Build history of the part. All positions in model axes, mm. Round coordinates to 2 decimals unless told otherwise and drop trailing zeros. Write each loop counter-clockwise with the first axis right and the second up, starting at its lowest first coordinate (ties: lowest second). Pieces come first, ordered by that corner, then holes. Notation, with made-up numbers: M 87,48 L 92,48 A14 ccw 92,59 Z; hole C 30,-32 d11. An arc over 180 degrees is marked long. Write item = value, one per line.
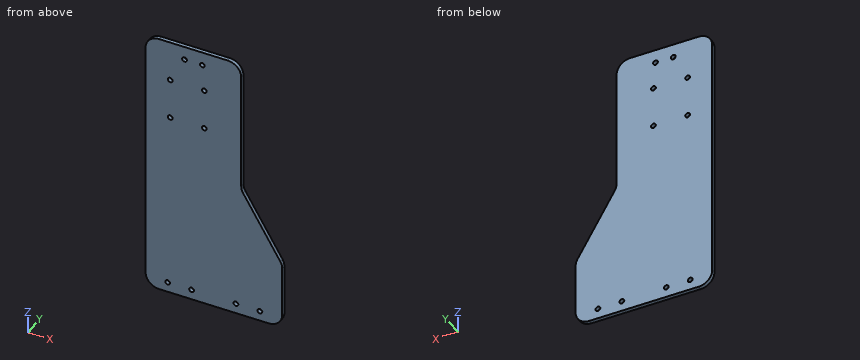
from build123d import *

# Parameters (mm, degrees)
SKETCH_1_W          = 100
SKETCH_1_H          = 200
EXTRUDE_1_DEPTH     = 3
CUT_EXTRUDE_1_DEPTH = 10
FILLET_2_R          = 10
SKETCH_4_R          = 1.75
CUT_EXTRUDE_2_DEPTH = 21
SKETCH_5_R          = 1.75
CUT_EXTRUDE_3_DEPTH = 4
SKETCH_7_R          = 1.75
CUT_EXTRUDE_4_DEPTH = 4


with BuildPart() as part:
    # 草图1 → 凸台-拉伸1 (new body)
    with BuildSketch(Plane(origin=(0, 0, 0), x_dir=(1, 0, 0), z_dir=(0, 1, 0))):
        Rectangle(SKETCH_1_W, SKETCH_1_H)
    extrude(amount=EXTRUDE_1_DEPTH)

    # 草图3 → 切除-拉伸1 (cut)
    with BuildSketch(Plane(origin=(0, 3, 0), x_dir=(1, 0, 0), z_dir=(0, 1, 0))):
        Polygon((20, -100), (20, 0), (50, 50), (50, -100), align=None)
    extrude(amount=-CUT_EXTRUDE_1_DEPTH, mode=Mode.SUBTRACT)

    # 圆角2
    fillet_2_edges = [part.edges().sort_by_distance(p)[0] for p in [
        (20, 1.5, 100),
        (20, 1.5, 0),
        (50, 1.5, -50),
        (-50, 1.5, 100),
        (-50, 1.5, -100),
        (50, 1.5, -100),
    ]]
    fillet(fillet_2_edges, radius=FILLET_2_R)

    # 草图4 → 切除-拉伸2 (cut)
    with BuildSketch(Plane(origin=(0, 3, 0), x_dir=(1, 0, 0), z_dir=(0, 1, 0))):
        with Locations(Location((33.647397187, 92.5, 0), (0, 0, 270))):
            Circle(SKETCH_4_R)
        with Locations(Location((16.132669012, 92.5, 0), (0, 0, 270))):
            Circle(SKETCH_4_R)
        with Locations(Location((-33.867330988, 92.5, 0), (0, 0, 270))):
            Circle(SKETCH_4_R)
        with Locations(Location((-16.352602813, 92.5, 0), (0, 0, 270))):
            Circle(SKETCH_4_R)
    extrude(amount=-CUT_EXTRUDE_2_DEPTH, mode=Mode.SUBTRACT)

    # 草图5 → 切除-拉伸3 (cut)
    with BuildSketch(Plane.XZ):
        with Locations(Location((-8.5, 90, 0), (0, 0, 270))):
            Circle(SKETCH_5_R)
        with Locations(Location((-21.5, 90, 0), (0, 0, 270))):
            Circle(SKETCH_5_R)
    extrude(amount=-CUT_EXTRUDE_3_DEPTH, mode=Mode.SUBTRACT)

    # 草图7 → 切除-拉伸4 (cut)
    with BuildSketch(Plane(origin=(0, 3, 0), x_dir=(1, 0, 0), z_dir=(0, 1, 0))):
        with Locations(Location((-32, -40, 0), (0, 0, 270))):
            Circle(SKETCH_7_R)
        with Locations(Location((-7, -40, 0), (0, 0, 270))):
            Circle(SKETCH_7_R)
        with Locations(Location((-7, -70, 0), (0, 0, 90))):
            Circle(SKETCH_7_R)
        with Locations(Location((-32, -70, 0), (0, 0, 90))):
            Circle(SKETCH_7_R)
    extrude(amount=-CUT_EXTRUDE_4_DEPTH, mode=Mode.SUBTRACT)


solid = part.part
1. Band-saw the part on A-A (y = 0.55). Count the separate pieces of the cut face and the enclosed holes in it, plus the area to 3 significant figures.
Responses:
separate_pieces = 1
enclosed_holes = 10
area = 16,100 mm²
2. Band-saw the part on B-B (z = -44). List the corners of the cut face in (x, y).
Responses:
outline = M -50,0 L 46.4,0 L 46.4,3 L -50,3 Z
3. Flat gauge pins, fed straight in: pin 1 (3 mm diameter, centred on x = -8.5, z = 90, fed in from +Y); pin 2 (5.5 mm diameter, centred on x = -7, z = 40, fed in from +Y); pin 3 (1.5 mm diameter, centred on y = 2, z = 61.5, fed in from +X). Where does each tip first touch, or does it go through?
Responses:
pin_1 = through
pin_2 = 3
pin_3 = 20
4. Band-saw the part on C-C (z = 14). List the corners of the cut face in (x, y).
Responses:
outline = M -50,0 L 20,0 L 20,3 L -50,3 Z
5. Probe probe 1 along X at (y, z) = (1.2, 70); probe 2 along X at (y, z) = (1.5, -92.5); probe 3 along X at (y, z) = (2.6, 58). List the from-to ranges inside material, lowest first.
Responses:
probe_1 = -50 to -33.75, -30.25 to -8.75, -5.25 to 20
probe_2 = -49.68 to -35.62, -32.12 to -18.1, -14.6 to 14.38, 17.88 to 31.9, 35.4 to 49.68
probe_3 = -50 to 20
